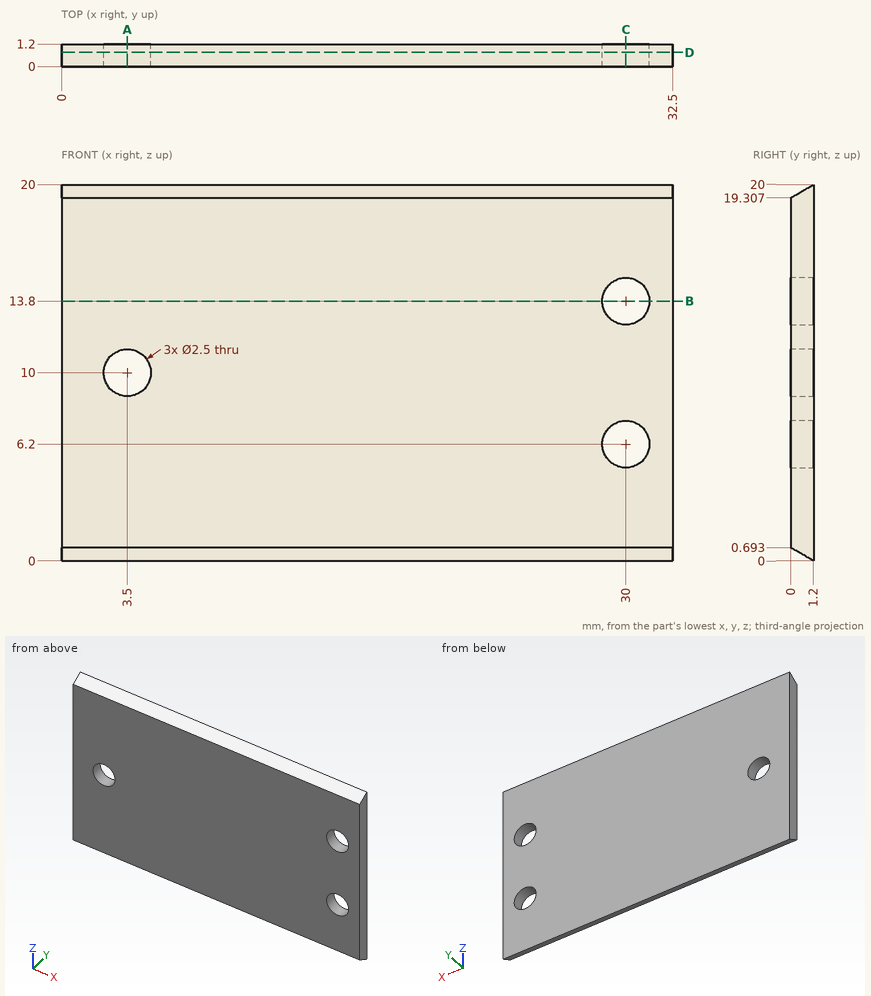
Verification items for this drawing (mm, ordinates from the low corner). Round coordinates to 2 decimals unless told otherwise and drop trailing zeros. Write each loop counter-clockwise with the first axis right and the second up, starting at its lowest first coordinate (ties: lowest second). Pieces come first, ordered by that corner, then holes. Notation, with made-up numbers: M -14,27 L -6,27 A31 cw -6,51 Z; hole C 21,87.5 d8. An arc over 180 degrees is marked long. Write item = value, one per line. Start each with the question number.
1. Section check A-A, the plane x = 3.5. Record the cut outline in (y, z), then the cut area to 3 significant figures.
2. Scan lines: line 1 (X direction, y = 0.75, z = 13.8); line 2 (X direction, y = 0.6, z = 10); line 3 (Z direction, x = 3, y = 0.5) (1 decimal). Record each from-to range of solid material in increasing order. Write a range as [from, to].
3. Section check B-B, the plane z = 13.8. Record the cut outline in (x, y).
4. Section check D-D, the plane y = 0.75. Record the cut outline in (x, z), then the cut area to 3 significant figures.
5. Section check C-C, the plane x = 30. Record the cut outline in (y, z).
Results found:
q1.outline = M 0,0.69 L 1.2,0 L 1.2,8.75 L 0,8.75 Z; M 0,11.25 L 1.2,11.25 L 1.2,20 L 0,19.31 Z
q1.area = 20.2 mm^2
q2.line_1 = [0, 28.75], [31.25, 32.5]
q2.line_2 = [0, 2.25], [4.75, 32.5]
q2.line_3 = [0.4, 8.9], [11.1, 19.6]
q3.outline = M 0,0 L 28.75,0 L 28.75,1.2 L 0,1.2 Z; M 31.25,0 L 32.5,0 L 32.5,1.2 L 31.25,1.2 Z
q4.outline = M 0,0.26 L 32.5,0.26 L 32.5,19.74 L 0,19.74 Z; hole C 3.5,10 d2.5; hole C 30,6.2 d2.5; hole C 30,13.8 d2.5
q4.area = 618 mm^2
q5.outline = M 0,0.69 L 1.2,0 L 1.2,4.95 L 0,4.95 Z; M 0,7.45 L 1.2,7.45 L 1.2,12.55 L 0,12.55 Z; M 0,15.05 L 1.2,15.05 L 1.2,20 L 0,19.31 Z
